from build123d import *

# Parameters (mm, degrees)
EXTRUDE_4_DEPTH  = 70
SKETCH_4_3_W     = 24
SKETCH_4_3_H     = 19
EXTRUDE_5_DEPTH  = 48
SKETCH_4_4_W     = 31
SKETCH_4_4_H     = 30
EXTRUDE_6_DEPTH  = 40
EXTRUDE_7_DEPTH  = 15
EXTRUDE_8_DEPTH  = 62
EXTRUDE_9_DEPTH  = 24
EXTRUDE_10_DEPTH = 86


with BuildPart() as part:
    # 스케치4 → 보스-돌출4 (new body)
    with BuildSketch(Plane.XY):
        Polygon((-55, 0), (0, 0), (0, 47), (-31, 47), (-31, 40), (-31, 21), (-55, 21), align=None)
        Polygon((0, 47), (0, 0), (55, 0), (55, 21), (31, 21), (31, 40), (31, 47), align=None)
    extrude(amount=EXTRUDE_4_DEPTH)

    # 스케치4<3> → 보스-돌출5 (add)
    with BuildSketch(Plane.XY):
        with Locations((43, 30.5)):
            Rectangle(SKETCH_4_3_W, SKETCH_4_3_H)
        with Locations((-43, 30.5)):
            Rectangle(SKETCH_4_3_W, SKETCH_4_3_H)
    extrude(amount=EXTRUDE_5_DEPTH)

    # 스케치4<4> → 보스-돌출6 (add)
    with BuildSketch(Plane.XY):
        with Locations((-15.5, 62)):
            Rectangle(SKETCH_4_4_W, SKETCH_4_4_H)
        with Locations((15.5, 62)):
            Rectangle(SKETCH_4_4_W, SKETCH_4_4_H)
    extrude(amount=EXTRUDE_6_DEPTH)

    # 스케치4<5> → 보스-돌출7 (add)
    with BuildSketch(Plane.XY):
        Polygon((31, 40), (55, 40), (31, 77), (31, 47), align=None)
        Polygon((-31, 77), (-55, 40), (-31, 40), (-31, 47), align=None)
    extrude(amount=EXTRUDE_7_DEPTH)

    # 스케치6 → 보스-돌출8 (add)
    with BuildSketch(Plane(origin=(31, 0, 0), x_dir=(0, 0, -1), z_dir=(1, 0, 0))):
        Polygon((-40, 77), (-70, 47), (-40, 47), align=None)
    extrude(amount=-EXTRUDE_8_DEPTH)

    # 스케치6<3> → 보스-돌출9 (add)
    with BuildSketch(Plane(origin=(31, 0, 0), x_dir=(0, 0, -1), z_dir=(1, 0, 0))):
        Polygon((-48, 40), (-70, 21), (-48, 21), align=None)
    extrude(amount=EXTRUDE_9_DEPTH)

    # 스케치6<4> → 보스-돌출10 (add)
    with BuildSketch(Plane(origin=(31, 0, 0), x_dir=(0, 0, -1), z_dir=(1, 0, 0))):
        Polygon((-48, 40), (-70, 21), (-48, 21), align=None)
    extrude(amount=-EXTRUDE_10_DEPTH)


solid = part.part
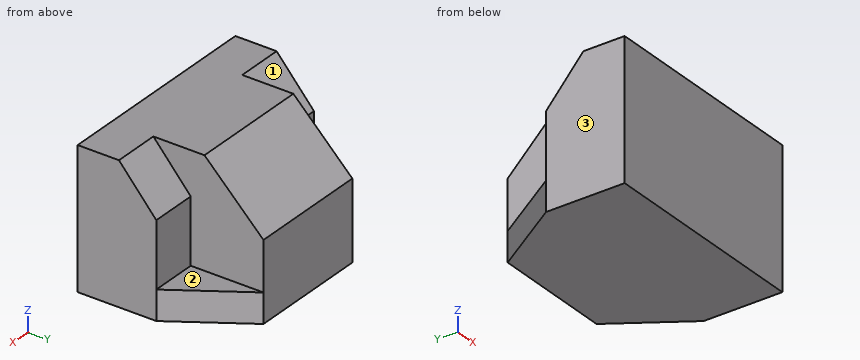
Can you work these out from the model? Positions are in its coordinate system, mm. Face numbers are marked on the shaded views. A direction names the side the tool comes from. Round coordinates to 2 decimals unless told otherwise and drop trailing zeros. Loops run counter-clockwise (first coordinate to the right, second up) from the corner with the lowest first, then second, coordinate; pieces in that order, holes last. Notation, with made-up numbers: (61.25, -9.75) - (106.25, -9.75) arc R23 cw to (106.25, 23.25) - close; hole circle Ø6 at (-2.5, 12). An arc over 180 degrees is marked (long way). Write item = value, one per line. Start each with the question number.
(1) If I drill on probe 1 along X at (y, z) = (74, 24); probe 2 along Y at (x, z) = (-36.5, 22.5); probe 3 along Z at (x, y) = (32, 43), over which ranges is the centre line in solid material (lowest first)? Write a range as [from, to].
(2) If we section it at A-A (z = 45): Please give me the cut outline in (x, y).
(3) For the marked faces 1, 2 and 3, which set-ups out of +Z, -Z, +X, -X, +Y, -Y let a thin tool reach every point of the face, with its end or its side?
(4) If we section it at B-B (x = -12.5): Please give me the cut outline in (y, z).
(5) For P1, Ø19, axis at x = -46, z = 29, coming from the +Y side; P2, Ø8, axis at x = -39, z = 13.5, coming from the +Y side; P3, Ø19, axis at x = 47, y = 60, coming from the +Z side, each with a flat end and sliding along its axis, tell me the tip position at first contact or that it passes through.
(6) If we section it at D-D (x = 48): Please give me the cut outline in (y, z), and give its area (3 significant figures).
(7) If we section it at C-C (y = 60.5): Please give me the cut outline in (x, z), and give its area (3 significant figures).
Ans:
q1.probe_1 = [-31, 31]
q1.probe_2 = [0, 40]
q1.probe_3 = [0, 15]
q2.outline = (-55, 0) - (55, 0) - (55, 40) - (31, 40) - (31, 72) - (-31, 72) - (-31, 40) - (-55, 40) - close
q3.face_1 = +Z, -X, +Y
q3.face_2 = +Z, +X, +Y
q3.face_3 = +Z, -Z, -X, +Y, -Y
q4.outline = (0, 0) - (77, 0) - (77, 40) - (47, 70) - (0, 70) - close
q5.P1 = 40
q5.P2 = 70.83
q5.P3 = 15
q6.outline = (0, 0) - (50.79, 0) - (50.79, 15) - (40, 15) - (40, 48) - (21, 70) - (0, 70) - close
q6.area = 2,750 mm²
q7.outline = (-41.7, 0) - (41.7, 0) - (41.7, 15) - (31, 15) - (31, 56.5) - (-31, 56.5) - (-31, 15) - (-41.7, 15) - close
q7.area = 3,820 mm²
